from build123d import *

# Parameters (mm, degrees)
SKETCH1_R           = 1.7
BOSS_EXTRUDE1_DEPTH = 6
FILLET1_R           = 1


with BuildPart() as part:
    # Sketch1 → Boss-Extrude1 (new body)
    # profile 1 of 2: a face of its own
    with BuildSketch(Plane.XY):
        with BuildLine():
            Line((10.5, -20.5), (-10.5, -20.5))
            Line((-10.5, -20.5), (-10.5, 20.5))
            Line((-10.5, 20.5), (10.5, 20.5))
            Line((10.5, 20.5), (10.5, 30.5))
            add(Edge.make_bspline(
                [(10.5, 30.5), (-5.463373434, 29.901564355), (-16.430762864, 42.802630452)],
                knots=[0, 0, 0, 1, 1, 1], degree=2))
            add(Edge.make_bspline(
                [(-16.430762864, 42.802630452), (-14.784114241, 25.00850842), (-28.192589157, 14.474851635)],
                knots=[0, 0, 0, 1, 1, 1], degree=2))
            add(Edge.make_bspline(
                [(-28.192589157, 14.474851635), (-25.736030858, -44.983019262), (-4.860661097, -100.922166241)],
                knots=[0, 0, 0, 0.989904815, 0.989904815, 0.989904815], degree=2))
            ThreePointArc((-4.860661097, -100.922166241), (-1.370198617, -94.941408132), (4.748458048, -98.184066997))
            add(Edge.make_bspline(
                [(12.954080919, -30.194198618), (-0.768915938, -62.557526438), (4.748458048, -98.184066997)],
                knots=[0, 0, 0, 0.978516684, 0.978516684, 0.978516684], degree=2))
            Line((12.954080919, -30.194198618), (10.5, -20.5))
        make_face()
        with Locations((-5, -24)):
            Circle(SKETCH1_R, mode=Mode.SUBTRACT)
        with Locations((5, -24)):
            Circle(SKETCH1_R, mode=Mode.SUBTRACT)
        with Locations((-5, 24)):
            Circle(SKETCH1_R, mode=Mode.SUBTRACT)
        with Locations((5, 24)):
            Circle(SKETCH1_R, mode=Mode.SUBTRACT)
    # profile 2 of 2: a face of its own
    with BuildSketch(Plane.XY):
        with BuildLine():
            add(Edge.make_bspline(
                [(4.748458048, -98.184066997), (4.86959189, -98.96624703), (5, -99.75)],
                knots=[0.978516684, 0.978516684, 0.978516684, 1, 1, 1], degree=2))
            ThreePointArc((4.748458048, -98.184066997), (-1.370198617, -94.941408132), (-4.860661097, -100.922166241))
            add(Edge.make_bspline(
                [(-4.860661097, -100.922166241), (-4.647771209, -101.492641346), (-4.432965727, -102.062750497)],
                knots=[0.989904815, 0.989904815, 0.989904815, 1, 1, 1], degree=2))
            ThreePointArc((-4.432965727, -102.062750497), (1.190624073, -104.606172806), (5, -99.75))
        make_face()
    extrude(amount=BOSS_EXTRUDE1_DEPTH)

    # Fillet1
    fillet1_edges = [part.edges().sort_by_distance(p)[0] for p in [
        (-28.192589157, 14.474851635, 3),
        (-16.430762864, 42.802630452, 3),
        (12.954080919, -30.194198618, 3),
    ]]
    fillet(fillet1_edges, radius=FILLET1_R)


solid = part.part
Can you work these out from the model? Positions are in its coordinate system, mm. A direction names the side the tool comes from. Coordinates: 2 decimals unless noted, no trailing zeros. Write item = value, one per line.
(1) Thinking about a two-plate mould opening in X: for faces 1 (the face through (-5.221, -22.314, 2.958)), 2 (the face through (-7, -31, 6)), 3 (the face through (5.914, -22.567, 2.958)), 4 (the face through (1.1, -104.628, 2.958)), which applies, +X half, -X half, draft (parallel to the pull), parting line (faces both ways), or undercut?
Verdict:
face_1 = undercut
face_2 = draft
face_3 = undercut
face_4 = parting line
(2) If I drill on probe 1 along Y at (x, z) = (2, 1.25); probe 2 along Y at (x, z) = (0, 2.75); probe 3 along X at (y, z) = (-90.5, 1.75), over which ranges is the centre line in solid material (lowest first)?
Verdict:
probe_1 = -104.33 to -20.5, 20.5 to 31.21
probe_2 = -104.75 to -20.5, 20.5 to 31.72
probe_3 = -8.58 to 3.78
(3) Imagine slicing it at A-A (y = -24). State how many separate pieces and enclosed holes the cut face has, and give its area (3 significant figures).
Verdict:
separate_pieces = 3
enclosed_holes = 0
area = 175 mm^2
(4) On a 3-axis mill with a long thin cutter (end or side, diameter ignored), from which of +Z, -Z, +X, -X, +Y, -Y can I reach the whole of each face in a straight line? I mean faces 5 (the face through (-7, -31, 0)), 6 (the face through (10.5, 25, 3)), 7 (the face through (-10.5, 0, 3)). Say none if no direction works.
Verdict:
face_5 = -Z, +X, -X, +Y, -Y
face_6 = +Z, -Z, +X, +Y
face_7 = +Z, -Z, +X
(5) For pin 1 (2 mm diameter, centred on x = 5, y = 24, fed in from +Z); pin 2 (1.5 mm diameter, centred on x = 4.5, z = 3, fed in from -Y); pin 3 (3 mm diameter, centred on x = 1, z = 4.5, fed in from +Y); pin 4 (3 mm diameter, centred on x = 4.5, z = 2.5, fed in from +Y), each with a flat end and sliding along its axis, tell me the tip position at first contact or that it passes through.
Verdict:
pin_1 = through
pin_2 = -103.06
pin_3 = 31.87
pin_4 = 31.01
